Read the model definition and answer for the solid it produces. Units are mm, in the model's axes. A direction names the side the tool comes from. Give positions to 0.01 mm unless a question says otherwise; leave off trailing zeros. Order: outer loops, then holes, each group sorted by start corner. A loop starts at its lowest first (then second) coordinate and runs counter-clockwise, first axis right, second up. Notation, with made-up numbers: M -12,13 L 12,13 A14 cw 12,17 Z; hole C -37.75,73 d3. An arc over 180 degrees is marked long. One line per item, written item: value. Start each with the question number.
from build123d import *

# Parameters (mm, degrees)
SKETCH_1_W                       = 40
SKETCH_1_H                       = 90
EXTRUDE_1_DEPTH                  = 40
SKETCH_2_W                       = 200
SKETCH_2_H                       = 200
EXTRUDE_2_DEPTH                  = 180
FILLET_3_R                       = 34
SHELL_5_T                        = -4
SKETCH_5_W                       = 32
SKETCH_5_H                       = 82
CUT_EXTRUDE_3_DEPTH              = 18
SKETCH_6_W                       = 20
SKETCH_6_H                       = 20
EXTRUDE_3_DEPTH                  = 360
SKETCH_7_W                       = 21
SKETCH_7_H                       = 21
EXTRUDE_4_DEPTH                  = 180
PATTERN_LINEAR_1_COUNT           = 2
PATTERN_LINEAR_1_PITCH           = 171
PATTERN_LINEAR_2_COUNT           = 2
PATTERN_LINEAR_2_PITCH           = 171
PATTERN_LINEAR_2_COPY_1_SKETCH_W = 20
PATTERN_LINEAR_2_COPY_1_SKETCH_H = 20
PATTERN_LINEAR_2_COPY_1_DEPTH    = 360
PATTERN_LINEAR_2_COPY_2_SKETCH_W = 21
PATTERN_LINEAR_2_COPY_2_SKETCH_H = 21
PATTERN_LINEAR_2_COPY_2_DEPTH    = 180
EXTRUDE_START                    = 30
SKETCH_8_W                       = 10
SKETCH_8_H                       = 50
EXTRUDE_8_DEPTH                  = 30
SKETCH_11_W                      = 10
SKETCH_11_H                      = 50
EXTRUDE_9_DEPTH                  = 30
SKETCH_12_R                      = 4.01
CUT_EXTRUDE_4_DEPTH              = 10
EXTRUDE_10_REACH                 = 402.78
SKETCH_18_W                      = 9
SKETCH_18_H                      = 21
CUT_EXTRUDE_5_DEPTH              = 170
SKETCH_20_W                      = 32.66
SKETCH_20_H                      = 47.99
CUT_EXTRUDE_6_DEPTH              = 20
SKETCH_21_R                      = 7.5
CUT_EXTRUDE_7_DEPTH              = 260


with BuildPart() as part:
    # 草图1 → 凸台-拉伸1 (new body)
    with BuildSketch(Plane.XY):
        with Locations((0, 45)):
            Rectangle(SKETCH_1_W, SKETCH_1_H)
    extrude(amount=EXTRUDE_1_DEPTH)

    # 草图2 → 凸台-拉伸2 (add)
    with BuildSketch(Plane.XY.offset(40)):
        with Locations((0, 45)):
            Rectangle(SKETCH_2_W, SKETCH_2_H)
    extrude(amount=EXTRUDE_2_DEPTH)

    # 圆角3
    fillet_3_edges = [part.edges().sort_by_distance(p)[0] for p in [
        (20, 45, 40),
        (0, 90, 40),
        (-20, 45, 40),
        (0, 0, 40),
    ]]
    fillet(fillet_3_edges, radius=FILLET_3_R)

    # 抽壳5
    shell_5_openings = [part.faces().sort_by_distance(p)[0] for p in [
        (0, 45, 220),
    ]]
    offset(amount=SHELL_5_T, openings=shell_5_openings)

    # 草图5 → 切除-拉伸3 (cut)
    with BuildSketch(Plane.XY.offset(4)):
        with Locations((0, 45)):
            Rectangle(SKETCH_5_W, SKETCH_5_H)
    extrude(amount=-CUT_EXTRUDE_3_DEPTH, mode=Mode.SUBTRACT)

    # 草图6 → 凸台-拉伸3 (add)
    with BuildSketch(Plane.XY.offset(220)):
        with Locations((-85, 130)):
            Rectangle(SKETCH_6_W, SKETCH_6_H)
    extrude_3 = extrude(amount=-EXTRUDE_3_DEPTH)

    # 草图7 → 凸台-拉伸4 (add)
    with BuildSketch(Plane.XY.offset(220)):
        with Locations((-85.5, 130.5)):
            Rectangle(SKETCH_7_W, SKETCH_7_H)
    extrude_4 = extrude(amount=-EXTRUDE_4_DEPTH)

    # 阵列(线性)1: 凸台-拉伸3, 凸台-拉伸4 ×2
    with Locations(*[(i * PATTERN_LINEAR_1_PITCH, 0, 0) for i in range(1, PATTERN_LINEAR_1_COUNT)]):
        add(extrude_3)
        add(extrude_4)

    # 阵列(线性)2: 凸台-拉伸3, 凸台-拉伸4 ×2
    with Locations(*[(0, -i * PATTERN_LINEAR_2_PITCH, 0) for i in range(1, PATTERN_LINEAR_2_COUNT)]):
        add(extrude_3)
        add(extrude_4)

    # 阵列(线性)2 copy 1 sketch → 阵列(线性)2 copy 1 (add)
    with BuildSketch(Plane(origin=(171, -171, 220), x_dir=(1, 0, 0), z_dir=(0, 0, 1))):
        with Locations((-85, 130)):
            Rectangle(PATTERN_LINEAR_2_COPY_1_SKETCH_W, PATTERN_LINEAR_2_COPY_1_SKETCH_H)
    extrude(amount=-PATTERN_LINEAR_2_COPY_1_DEPTH)

    # 阵列(线性)2 copy 2 sketch → 阵列(线性)2 copy 2 (add)
    with BuildSketch(Plane(origin=(171, -171, 220), x_dir=(1, 0, 0), z_dir=(0, 0, 1))):
        with Locations((-85.5, 130.5)):
            Rectangle(PATTERN_LINEAR_2_COPY_2_SKETCH_W, PATTERN_LINEAR_2_COPY_2_SKETCH_H)
    extrude(amount=-PATTERN_LINEAR_2_COPY_2_DEPTH)

    # 草图8 → 凸台-拉伸8 (add)
    with BuildSketch(Plane.ZY.offset(20).offset(EXTRUDE_START)):
        with Locations((5, 45.224395516)):
            Rectangle(SKETCH_8_W, SKETCH_8_H)
    extrude(amount=-EXTRUDE_8_DEPTH)

    # 草图11 → 凸台-拉伸9 (add)
    with BuildSketch(Plane(origin=(20, 0, 0), x_dir=(0, 0, -1), z_dir=(1, 0, 0))):
        with Locations((-5, 45)):
            Rectangle(SKETCH_11_W, SKETCH_11_H)
    extrude(amount=EXTRUDE_9_DEPTH)

    # 草图12 → 切除-拉伸4 (cut)
    with BuildSketch(Plane(origin=(0, 0, 0), x_dir=(-1, 0, 0), z_dir=(0, 0, -1))):
        with Locations((-35, 45.224395516)):
            Circle(SKETCH_12_R)
        with Locations((35, 45.224395516)):
            Circle(SKETCH_12_R)
    extrude(amount=-CUT_EXTRUDE_4_DEPTH, mode=Mode.SUBTRACT)

    # 草图17 → 凸台-拉伸10 (add, up to next)
    with BuildSketch(Plane.XY.offset(220), mode=Mode.PRIVATE) as extrude_10_sk1:
        Polygon((-75, 120), (75, 120), (96, 120), (96, 115), (-96, 115), (-96, 120), align=None)
    extrude_10_tool1 = extrude(extrude_10_sk1.sketch, amount=-EXTRUDE_10_REACH, mode=Mode.PRIVATE) - part.part
    add(extrude_10_tool1.solids().sort_by_distance((0, 117.5, 220))[0])

    # 草图18 → 切除-拉伸5 (cut)
    with BuildSketch(Plane.XY.offset(220)):
        with Locations((79.5, 130.5)):
            Rectangle(SKETCH_18_W, SKETCH_18_H)
        with Locations((-79.5, 130.5)):
            Rectangle(SKETCH_18_W, SKETCH_18_H)
    extrude(amount=-CUT_EXTRUDE_5_DEPTH, mode=Mode.SUBTRACT)

    # 草图20 → 切除-拉伸6 (cut)
    with BuildSketch(Plane(origin=(0, 145, 0), x_dir=(1, 0, 0), z_dir=(0, 1, 0))):
        with Locations((0, -106.354128517)):
            Rectangle(SKETCH_20_W, SKETCH_20_H)
    extrude(amount=-CUT_EXTRUDE_6_DEPTH, mode=Mode.SUBTRACT)

    # 草图21 → 切除-拉伸7 (cut)
    with BuildSketch(Plane(origin=(0, 0, 40), x_dir=(-1, 0, 0), z_dir=(0, 0, -1))):
        with Locations(Location((0, 131, 0), (0, 0, 291.039469781))):
            Circle(SKETCH_21_R)
    extrude(amount=-CUT_EXTRUDE_7_DEPTH, mode=Mode.SUBTRACT)


solid = part.part
Q1. Consider probe 1 along Y at (x, z) = (-25, 93.5); probe 2 along X at (y, z) = (8, 123.5); probe 3 along X at (y, z) = (131, 41.2). Determine where each line is inside the solid, lowest interval first.
Q2. Find section A-A, the plane y = 29.5. Give the vertices of the cut face in (x, z), then the cut area to 3 significant figures.
Q3. Find section D-D, the plane z = 20. Give the vertices of the cut face in (x, y), then the cut area to 3 significant figures.
Q4. Each of these flat-tipped pins is pushed along its axis until it touches: pin 1 (3 mm diameter, centred on x = -6.5, z = 4, fed in from +Y); pin 2 (4 mm diameter, centred on x = -21, y = 58.5, fed in from +Z); pin 3 (1 mm diameter, centred on x = -75.5, z = -8, fed in from -Y). Where does it stop, or does it pass through?
Q5. A tool of negligible diameter and unlimited length cuts with its end or side. For faces 1 (the flat face through (-35, 70.224, 5)), 2 (the flat face through (-85, 120, -49)), 3 (the cylindrical face through (0.756, -12.548, 37.366)), 4 (the cylindrical face through (0.756, -14.806, 34.064)), 5 (the flat face through (-85, -51, -49)), from which of +Z, -Z, +X, -X, +Y, -Y can it reach the whole face along a straight path? Write none if from no direction.
Q6. Find section B-B, the plane z = 65.5. Give the vertices of the cut face in (x, y), then the cut area to 3 significant figures.
Q7. Find section C-C, the plane z = -47.5. Give the vertices of the cut face in (x, y), then the cut area to 3 significant figures.
Q8. Determine the mould class of faces 6 (the flat face through (86, -31, -49)), 7 (the flat face through (100, 44, 129)), 8 (the cylindrical face through (32.548, 41.543, 37.366)), 9 (the flat face through (-75, 130, -49)) for opening direction X: released by +X, released by -X, zero draft, split by the parting line, or undercut.
Evaluation:
1. probe 1: -55 to -51, 115 to 120, 141 to 145
1. probe 2: -100 to -96, 96 to 100
1. probe 3: -100 to -7.5, 7.5 to 100
2. outline: M -100,40 L -54,40 A34 cw -20.24,10 L -50,10 L -50,0 L -16,0 L -16,6 A38 ccw -54,44 L -96,44 L -96,220 L -100,220 Z; M 16,0 L 50,0 L 50,10 L 20.24,10 A34 cw 54,40 L 100,40 L 100,220 L 96,220 L 96,44 L 54,44 A38 ccw 16,6 Z
2. area: 2,880 mm2
3. outline: M -95,-51 L -75,-51 L -75,-31 L -95,-31 Z; M -95,120 L -75,120 L -75,140 L -95,140 Z; M -23.02,-3.02 L 23.02,-3.02 L 23.02,93.02 L -23.02,93.02 Z; M 76,-51 L 96,-51 L 96,-31 L 76,-31 Z; M 76,120 L 96,120 L 96,140 L 76,140 Z; hole M -18.67,1.33 L 18.67,1.33 L 18.67,88.67 L -18.67,88.67 Z
3. area: 2,760 mm2
4. pin 1: y = 90
4. pin 2: z = 27.98
4. pin 3: y = -51
5. face 1: -Z, -X, +Y
5. face 2: -Z, +X, -X
5. face 3: +Z
5. face 4: -Z, -Y
5. face 5: -Z, +X, -X, -Y
6. outline: M -100,-55 L 100,-55 L 100,145 L -100,145 Z; hole M -96,-30 L -75,-30 L -75,-51 L 75,-51 L 75,-30 L 96,-30 L 96,115 L -96,115 Z; hole M -84,120 L 84,120 L 84,141 L -84,141 Z
6. area: 5,480 mm2
7. outline: M -95,-51 L -75,-51 L -75,-31 L -95,-31 Z; M -95,120 L -75,120 L -75,140 L -95,140 Z; M 76,-51 L 96,-51 L 96,-31 L 76,-31 Z; M 76,120 L 96,120 L 96,140 L 76,140 Z
7. area: 1,600 mm2
8. face 6: zero draft
8. face 7: released by +X
8. face 8: undercut
8. face 9: undercut
